from build123d import *

# Parameters (mm, degrees)
F0_W     = 278.4
F0_H     = 224.4
F1_DEPTH = 57.5
F2_R     = 61.2
F3_T     = -1.2
F5_DEPTH = 1.2
F6_R     = 2
F7_R     = 1.5
F8_DEPTH = 1.2


# Not quite as in the source:
# - a feature names something its author has since deleted; it is built from what else it names


with BuildPart() as f1:
    # F0 (on Top) → F1 (new body, symmetric)
    with BuildSketch(Plane.XY):
        Rectangle(F0_W, F0_H)
    extrude(amount=F1_DEPTH, both=True)

    # F2
    f2_edges = [f1.edges().sort_by_distance(p)[0] for p in [
        (-139.2, -112.2, 0),
        (139.2, -112.2, 0),
        (139.2, 112.2, 0),
        (-139.2, 112.2, 0),
    ]]
    fillet(f2_edges, radius=F2_R)

    # F3
    f3_openings = [f1.faces().sort_by_distance(p)[0] for p in [
        (0, 0, 57.5),
    ]]
    offset(amount=F3_T, openings=f3_openings)

    # F4 (on face) → F5 (join)
    with BuildSketch(Plane.XY.offset(57.5)):
        with BuildLine():
            ThreePointArc((-163, -51), (-138.1040764009, -111.1040764009), (-78, -136))
            Line((-78, -136), (78, -136))
            ThreePointArc((78, -136), (138.1040764009, -111.1040764009), (163, -51))
            Line((163, -51), (163, 51))
            ThreePointArc((163, 51), (138.1040764009, 111.1040764009), (78, 136))
            Line((78, 136), (-78, 136))
            ThreePointArc((-78, 136), (-138.1040764009, 111.1040764009), (-163, 51))
            Line((-163, 51), (-163, -51))
        make_face()
        with BuildLine():
            ThreePointArc((138, -51), (120.4264068712, -93.4264068712), (78, -111))
            Line((78, -111), (-78, -111))
            ThreePointArc((-78, -111), (-120.4264068712, -93.4264068712), (-138, -51))
            Line((-138, -51), (-138, 51))
            ThreePointArc((-138, 51), (-120.4264068712, 93.4264068712), (-78, 111))
            Line((-78, 111), (78, 111))
            ThreePointArc((78, 111), (120.4264068712, 93.4264068712), (138, 51))
            Line((138, 51), (138, -51))
        make_face(mode=Mode.SUBTRACT)
    extrude(amount=F5_DEPTH)

    # F6
    f6_edges = [f1.edges().sort_by_distance(p)[0] for p in [
        (0, -112.2, -57.5),
        (139.2, 0, -57.5),
        (0, 112.2, -57.5),
        (-139.2, 0, -57.5),
        (-121.274935, -94.274935, -57.5),
        (-121.274935, 94.274935, -57.5),
        (121.274935, 94.274935, -57.5),
        (121.274935, -94.274935, -57.5),
    ]]
    fillet(f6_edges, radius=F6_R)

    # F7 (on face) → F8 (cut, through all)
    with BuildSketch(Plane.XY.offset(-56.3)):
        with Locations((-111.7, 86)):
            Circle(F7_R)
        with Locations((-111.7, 61)):
            Circle(F7_R)
        with Locations((-111.7, 36)):
            Circle(F7_R)
        with Locations((-111.7, 11)):
            Circle(F7_R)
        with Locations((-111.7, -14)):
            Circle(F7_R)
        with Locations((-111.7, -39)):
            Circle(F7_R)
        with Locations((-111.7, -64)):
            Circle(F7_R)
        with Locations((-111.7, -89)):
            Circle(F7_R)
        with Locations((-86.7, 86)):
            Circle(F7_R)
        with Locations((-86.7, 61)):
            Circle(F7_R)
        with Locations((-86.7, 36)):
            Circle(F7_R)
        with Locations((-86.7, 11)):
            Circle(F7_R)
        with Locations((-86.7, -14)):
            Circle(F7_R)
        with Locations((-86.7, -39)):
            Circle(F7_R)
        with Locations((-86.7, -64)):
            Circle(F7_R)
        with Locations((-86.7, -89)):
            Circle(F7_R)
        with Locations((-61.7, 86)):
            Circle(F7_R)
        with Locations((-61.7, 61)):
            Circle(F7_R)
        with Locations((-61.7, 36)):
            Circle(F7_R)
        with Locations((-61.7, 11)):
            Circle(F7_R)
        with Locations((-61.7, -14)):
            Circle(F7_R)
        with Locations((-61.7, -39)):
            Circle(F7_R)
        with Locations((-61.7, -64)):
            Circle(F7_R)
        with Locations((-61.7, -89)):
            Circle(F7_R)
        with Locations((-36.7, 86)):
            Circle(F7_R)
        with Locations((-36.7, 61)):
            Circle(F7_R)
        with Locations((-36.7, 36)):
            Circle(F7_R)
        with Locations((-36.7, 11)):
            Circle(F7_R)
        with Locations((-36.7, -14)):
            Circle(F7_R)
        with Locations((-36.7, -39)):
            Circle(F7_R)
        with Locations((-36.7, -64)):
            Circle(F7_R)
        with Locations((-36.7, -89)):
            Circle(F7_R)
        with Locations((-11.7, 86)):
            Circle(F7_R)
        with Locations((-11.7, 61)):
            Circle(F7_R)
        with Locations((-11.7, 36)):
            Circle(F7_R)
        with Locations((-11.7, 11)):
            Circle(F7_R)
        with Locations((-11.7, -14)):
            Circle(F7_R)
        with Locations((-11.7, -39)):
            Circle(F7_R)
        with Locations((-11.7, -64)):
            Circle(F7_R)
        with Locations((-11.7, -89)):
            Circle(F7_R)
        with Locations((13.3, 86)):
            Circle(F7_R)
        with Locations((13.3, 61)):
            Circle(F7_R)
        with Locations((13.3, 36)):
            Circle(F7_R)
        with Locations((13.3, 11)):
            Circle(F7_R)
        with Locations((13.3, -14)):
            Circle(F7_R)
        with Locations((13.3, -39)):
            Circle(F7_R)
        with Locations((13.3, -64)):
            Circle(F7_R)
        with Locations((13.3, -89)):
            Circle(F7_R)
        with Locations((38.3, 86)):
            Circle(F7_R)
        with Locations((38.3, 61)):
            Circle(F7_R)
        with Locations((38.3, 36)):
            Circle(F7_R)
        with Locations((38.3, 11)):
            Circle(F7_R)
        with Locations((38.3, -14)):
            Circle(F7_R)
        with Locations((38.3, -39)):
            Circle(F7_R)
        with Locations((38.3, -64)):
            Circle(F7_R)
        with Locations((38.3, -89)):
            Circle(F7_R)
        with Locations((63.3, 86)):
            Circle(F7_R)
        with Locations((63.3, 61)):
            Circle(F7_R)
        with Locations((63.3, 36)):
            Circle(F7_R)
        with Locations((63.3, 11)):
            Circle(F7_R)
        with Locations((63.3, -14)):
            Circle(F7_R)
        with Locations((63.3, -39)):
            Circle(F7_R)
        with Locations((63.3, -64)):
            Circle(F7_R)
        with Locations((63.3, -89)):
            Circle(F7_R)
        with Locations((88.3, 86)):
            Circle(F7_R)
        with Locations((88.3, 61)):
            Circle(F7_R)
        with Locations((88.3, 36)):
            Circle(F7_R)
        with Locations((88.3, 11)):
            Circle(F7_R)
        with Locations((88.3, -14)):
            Circle(F7_R)
        with Locations((88.3, -39)):
            Circle(F7_R)
        with Locations((88.3, -64)):
            Circle(F7_R)
        with Locations((88.3, -89)):
            Circle(F7_R)
        with Locations((113.3, 86)):
            Circle(F7_R)
        with Locations((113.3, 61)):
            Circle(F7_R)
        with Locations((113.3, 36)):
            Circle(F7_R)
        with Locations((113.3, 11)):
            Circle(F7_R)
        with Locations((113.3, -14)):
            Circle(F7_R)
        with Locations((113.3, -39)):
            Circle(F7_R)
        with Locations((113.3, -64)):
            Circle(F7_R)
        with Locations((113.3, -89)):
            Circle(F7_R)
    extrude(amount=-F8_DEPTH, mode=Mode.SUBTRACT)


solid = f1.part
Can you work these out from the model? Positions are in its coordinate system, mm. A direction names the side the tool comes from. Give positions to 0.01 mm unless a question says otherwise; leave off trailing zeros. Order: outer loops, then holes, each group sorted by start corner. A loop starts at its lowest first (then second) coordinate and runs counter-clockwise, first axis right, second up. Notation, with made-up numbers: M 24,-5 L 41,-5 A33 cw 41,24 Z; hole C -18,25 d2. An arc over 180 degrees is marked long. One line per item, written item: value.
Item 1: If we section it at B-B on y = 28.5: Write out the boundary of the cut face in (x, z), and give its area (3 significant figures).
Verdict:
outline: M -163,57.5 L -139.2,57.5 L -139.2,-55.5 A2 ccw -137.2,-57.5 L 137.2,-57.5 A2 ccw 139.2,-55.5 L 139.2,57.5 L 163,57.5 L 163,58.7 L 138,58.7 L 138,-56.3 L -138,-56.3 L -138,58.7 L -163,58.7 Z
area: 665 mm2
Item 2: If we mould it in two halves opening along X, with no side actions, what happens to faces 4 (the face through (-12.8, 111.4, 58.7)), 5 (the face through (137.4, -111.8, 58.1)), 6 (the face through (138, 1, 0))? For each: pulls with the +X half, pulls with the -X half, needs draft (parallel to the pull), parting line crosses it, or undercut.
Verdict:
face 4: needs draft
face 5: pulls with the +X half
face 6: undercut
Item 3: For pin 1 (12 mm diameter, centred on y = -43.5, z = -27.5, fed in from -X); pin 2 (4 mm diameter, centred on x = 13.3, y = 61, fed in from +Z); pin 3 (6 mm diameter, centred on x = 5.5, z = -31.5, fed in from -Y), each with a flat end and sliding along its axis, tell me the tip position at first contact or that it passes through.
Verdict:
pin 1: x = -139.2
pin 2: z = -56.3
pin 3: y = -112.2
Item 4: Please list where these lines run through material, in increasing order: line 1 (X direction, y = -21.5, z = 50.5); line 2 (Y direction, x = -61, z = -56); line 3 (Y direction, x = -8.5, z = -35).
Verdict:
line 1: -139.2 to -138, 138 to 139.2
line 2: -112.14 to -111, 111 to 112.14
line 3: -112.2 to -111, 111 to 112.2
Item 5: For faces 1 (the face through (-2, 2, -56.3)), 2 (the face through (-1, -112.2, 2)), 3 (the face through (121.748, 93.796, 0.209)), which set-ups out of +Z, -Z, +X, -X, +Y, -Y let a thin tool reach every point of the face, with its end or its side?
Verdict:
face 1: +Z
face 2: -Z, +X, -X, -Y
face 3: -Z, +X, +Y
Item 6: If we section it at A-A on z = -38: Write out the boundary of the cut face in (x, y).
Verdict:
outline: M -139.2,-51 A61.2 ccw -78,-112.2 L 78,-112.2 A61.2 ccw 139.2,-51 L 139.2,51 A61.2 ccw 78,112.2 L -78,112.2 A61.2 ccw -139.2,51 Z; hole M -138,-51 A60 ccw -78,-111 L 78,-111 A60 ccw 138,-51 L 138,51 A60 ccw 78,111 L -78,111 A60 ccw -138,51 Z
